Geometry check sheet. Reference: the model listing, model coordinates, mm. A direction names the side the tool comes from. Give positions to 0.01 mm unless a question says otherwise; leave off trailing zeros. Write each loop counter-clockwise with the first axis right and the second up, starting at its lowest first coordinate (ties: lowest second). Pieces come first, ordered by that corner, then holes.
(1) Cross-section at C-C (y = -33.5). Record the boundary of the cut face in (x, z).
(2) Thickness scan on line 1 along Y through (x, z) = (28, 2.9); line 2 along X through (y, z) = (27, 2.2); line 3 along Y through (x, z) = (-0.5, 0.7). Record the ranges inside material, lowest first.
(3) Cross-section at A-A (y = 48). Record the boundary of the cut face in (x, z).
(4) Cross-section at B-B (x = 1). Record the boundary of the cut face in (y, z).
(5) Tool access check on faces 4 (the cylindrical face through (-29.1, 48.07, 2.59)), 5 (the cylindrical face through (26.64, -42.1, 2.19)), 6 (the flat face through (30.5, -48, 1)). Record the directions out of +Z, -Z, +X, -X, +Y, -Y that give a thin tool (end or side, any length) a straight path to the whole face; none if there is none.
(6) Depth check by flat-ended pin: P1, Ø1, axis at x = -8.5, z = 2.5, coming from the +Y side; P2, Ø4, axis at x = -9, y = 8, coming from the +Z side; P3, Ø1.8, axis at x = 27, y = -49.5, coming from the -Z side. Enter the tip coordinate at first touch or a pass-through.
(7) Mould release check, pull along X, two halves, no side actions. Record for faces 1 (the cylindrical face through (32.108, 52.776, 1.578)), 2 (the flat face through (0, -53, 2)), 3 (the flat face through (-29, -47, 2)): +X half, -X half, draft (parallel to the pull), parting line (faces both ways), or undercut.
```python
from build123d import *

# Parameters (mm, degrees)
F1_DEPTH = 3.2
F2_DEPTH = 1.2
F3_START = 2
F0_R     = 1.6
F3_DEPTH = 1.2


with BuildPart() as f1:
    # F0 (on Top) → F1 (new body)
    with BuildSketch(Plane.XY):
        with BuildLine():
            Line((-32.5, 51.2930130847), (-32.5, 48))
            Line((-32.5, 48), (-32.5, -48))
            Line((-32.5, -48), (-32.5, -50))
            ThreePointArc((-32.5, -50), (-31.6213203436, -52.1213203436), (-29.5, -53))
            Line((-29.5, -53), (29.5, -53))
            ThreePointArc((29.5, -53), (31.6213203436, -52.1213203436), (32.5, -50))
            Line((32.5, -50), (32.5, -48))
            Line((32.5, -48), (32.5, 48))
            Line((32.5, 48), (32.5, 51.2930130847))
            ThreePointArc((32.5, 51.2930130847), (32.0968235498, 52.7951806689), (30.9956616994, 53.8935891904))
            ThreePointArc((30.9956616994, 53.8935891904), (0, 62.1711347813), (-30.9956616994, 53.8935891904))
            ThreePointArc((-30.9956616994, 53.8935891904), (-32.0968235498, 52.7951806689), (-32.5, 51.2930130847))
        make_face()
        Polygon((-27.5, -44.5358983849), (-24.5, -46.2679491924), (-24.5, -49.7320508076), (-27.5, -51.4641016151), (-30.5, -49.7320508076), (-30.5, -46.2679491924), align=None, mode=Mode.SUBTRACT)
        Polygon((27.5, -51.4641016151), (24.5, -49.7320508076), (24.5, -46.2679491924), (27.5, -44.5358983849), (30.5, -46.2679491924), (30.5, -49.7320508076), align=None, mode=Mode.SUBTRACT)
        with BuildLine():
            ThreePointArc((-27.5, 40), (-26.6213203436, 42.1213203436), (-24.5, 43))
            Line((-24.5, 43), (24.5, 43))
            ThreePointArc((24.5, 43), (26.6213203436, 42.1213203436), (27.5, 40))
            Line((27.5, 40), (27.5, -40))
            ThreePointArc((27.5, -40), (26.6213203436, -42.1213203436), (24.5, -43))
            Line((24.5, -43), (-24.5, -43))
            ThreePointArc((-24.5, -43), (-26.6213203436, -42.1213203436), (-27.5, -40))
            Line((-27.5, -40), (-27.5, 40))
        make_face(mode=Mode.SUBTRACT)
        Polygon((-27.5, 51.4641016151), (-24.5, 49.7320508076), (-24.5, 46.2679491924), (-27.5, 44.5358983849), (-30.5, 46.2679491924), (-30.5, 49.7320508076), align=None, mode=Mode.SUBTRACT)
        with BuildLine():
            ThreePointArc((-7.4999998324, 55), (-9.4999998324, 57), (-7.4999998324, 59))
            Line((-7.4999998324, 59), (7.5000001676, 59))
            ThreePointArc((7.5000001676, 59), (9.5000001676, 57), (7.5000001676, 55))
            Line((7.5000001676, 55), (-7.4999998324, 55))
        make_face(mode=Mode.SUBTRACT)
        Polygon((27.5, 44.5358983849), (24.5, 46.2679491924), (24.5, 49.7320508076), (27.5, 51.4641016151), (30.5, 49.7320508076), (30.5, 46.2679491924), align=None, mode=Mode.SUBTRACT)
    extrude(amount=F1_DEPTH)

    # F0 (on Top) → F2 (join)
    with BuildSketch(Plane.XY):
        with BuildLine():
            Line((24.5, 43), (-24.5, 43))
            ThreePointArc((-24.5, 43), (-26.6213203436, 42.1213203436), (-27.5, 40))
            Line((-27.5, 40), (-27.5, -40))
            ThreePointArc((-27.5, -40), (-26.6213203436, -42.1213203436), (-24.5, -43))
            Line((-24.5, -43), (24.5, -43))
            ThreePointArc((24.5, -43), (26.6213203436, -42.1213203436), (27.5, -40))
            Line((27.5, -40), (27.5, 40))
            ThreePointArc((27.5, 40), (26.6213203436, 42.1213203436), (24.5, 43))
        make_face()
    extrude(amount=F2_DEPTH)

    # F0 (on Top) → F3 (join)
    with BuildSketch(Plane.XY.offset(F3_START)):
        Polygon((-24.5, -49.7320508076), (-24.5, -46.2679491924), (-27.5, -44.5358983849), (-30.5, -46.2679491924), (-30.5, -49.7320508076), (-27.5, -51.4641016151), align=None)
        with Locations((-27.5, -48)):
            Circle(F0_R, mode=Mode.SUBTRACT)
        Polygon((24.5, -46.2679491924), (24.5, -49.7320508076), (27.5, -51.4641016151), (30.5, -49.7320508076), (30.5, -46.2679491924), (27.5, -44.5358983849), align=None)
        with Locations((27.5, -48)):
            Circle(F0_R, mode=Mode.SUBTRACT)
        Polygon((24.5, 49.7320508076), (24.5, 46.2679491924), (27.5, 44.5358983849), (30.5, 46.2679491924), (30.5, 49.7320508076), (27.5, 51.4641016151), align=None)
        with Locations((27.5, 48)):
            Circle(F0_R, mode=Mode.SUBTRACT)
        Polygon((-24.5, 46.2679491924), (-24.5, 49.7320508076), (-27.5, 51.4641016151), (-30.5, 49.7320508076), (-30.5, 46.2679491924), (-27.5, 44.5358983849), align=None)
        with Locations((-27.5, 48)):
            Circle(F0_R, mode=Mode.SUBTRACT)
    extrude(amount=F3_DEPTH)


solid = f1.part
```
Reply:
1. outline: (-32.5, 0) - (32.5, 0) - (32.5, 3.2) - (27.5, 3.2) - (27.5, 1.2) - (-27.5, 1.2) - (-27.5, 3.2) - (-32.5, 3.2) - close
2. line 1: y = -53 to -49.52, -46.48 to 46.48, 49.52 to 55.51
2. line 2: x = -32.5 to -27.5, 27.5 to 32.5
2. line 3: y = -53 to 55, 59 to 62.17
3. outline: (-32.5, 0) - (-30.5, 0) - (-30.5, 2) - (-29.1, 2) - (-29.1, 3.2) - (-32.5, 3.2) - close; (-25.9, 2) - (-24.5, 2) - (-24.5, 0) - (24.5, 0) - (24.5, 2) - (25.9, 2) - (25.9, 3.2) - (-25.9, 3.2) - close; (29.1, 2) - (30.5, 2) - (30.5, 0) - (32.5, 0) - (32.5, 3.2) - (29.1, 3.2) - close
4. outline: (-53, 0) - (55, 0) - (55, 3.2) - (43, 3.2) - (43, 1.2) - (-43, 1.2) - (-43, 3.2) - (-53, 3.2) - close; (59, 0) - (62.16, 0) - (62.16, 3.2) - (59, 3.2) - close
5. face 4: +Z, -Z
5. face 5: +Z
5. face 6: -Z
6. P1: stops at y = 61.65
6. P2: stops at z = 1.2
6. P3: stops at z = 2
7. face 1: +X half
7. face 2: draft
7. face 3: undercut
